Verification items for the finished model (mm, model axes). A direction names the side the tool comes from. Give positions to 0.01 mm unless a question says otherwise; leave off trailing zeros. Write each loop counter-clockwise with the first axis right and the second up, starting at its lowest first coordinate (ties: lowest second). Pieces come first, ordered by that corner, then holes. Notation, with made-up numbers: (12, 15) -> (31, 15) arc R24 cw to (31, 46) -> close; hole circle Ø11 at (71.5, 18). An arc over 180 degrees is marked (long way). Write item = value, one per line.
from build123d import *

# Parameters (mm, degrees)
SKETCH1_W           = 1043.686
SKETCH1_H           = 730.25
BOSS_EXTRUDE1_DEPTH = 6.35
SKETCH9_W           = 304.8
SKETCH9_H           = 304.8
CUT_EXTRUDE3_DEPTH  = 6.35
CUT_EXTRUDE4_DEPTH  = 6.35
FILLET1_R           = 6.35
CUT_EXTRUDE6_DEPTH  = 7.35


with BuildPart() as part:
    # Sketch1 → Boss-Extrude1 (new body)
    with BuildSketch(Plane.XY):
        with Locations((521.843, 365.125)):
            Rectangle(SKETCH1_W, SKETCH1_H)
    extrude(amount=BOSS_EXTRUDE1_DEPTH)

    # Sketch9 → Cut-Extrude3 (cut)
    with BuildSketch(Plane(origin=(0, 0, 0), x_dir=(-1, 0, 0), z_dir=(0, 0, -1))):
        with Locations((-196.85, 228.6)):
            Rectangle(SKETCH9_W, SKETCH9_H)
    extrude(amount=-CUT_EXTRUDE3_DEPTH, mode=Mode.SUBTRACT)

    # Sketch10 → Cut-Extrude4 (cut)
    with BuildSketch(Plane.XY.offset(6.35)):
        with BuildLine():
            Line((76.2, 50.8), (0, 50.8))
            Line((0, 50.8), (0, 0))
            Line((0, 0), (101.6, 0))
            Line((101.6, 0), (101.6, 25.4))
            ThreePointArc((101.6, 25.4), (94.160512242, 43.360512242), (76.2, 50.8))
        make_face()
        with BuildLine():
            Line((942.086, 25.4), (942.086, 0))
            Line((942.086, 0), (1043.686, 0))
            Line((1043.686, 0), (1043.686, 50.8))
            Line((1043.686, 50.8), (967.486, 50.8))
            ThreePointArc((967.486, 50.8), (949.525487758, 43.360512242), (942.086, 25.4))
        make_face()
        with BuildLine():
            Line((967.486, 558.8), (1043.686, 558.8))
            Line((1043.686, 558.8), (1043.686, 476.25))
            Line((1043.686, 476.25), (967.486, 476.25))
            ThreePointArc((967.486, 476.25), (949.525487758, 483.689487758), (942.086, 501.65))
            Line((942.086, 501.65), (942.086, 533.4))
            ThreePointArc((942.086, 533.4), (949.525487758, 551.360512242), (967.486, 558.8))
        make_face()
        with BuildLine():
            Line((76.2, 558.8), (0, 558.8))
            Line((0, 558.8), (0, 476.25))
            Line((0, 476.25), (76.2, 476.25))
            ThreePointArc((76.2, 476.25), (94.160512242, 483.689487758), (101.6, 501.65))
            Line((101.6, 501.65), (101.6, 533.4))
            ThreePointArc((101.6, 533.4), (94.160512242, 551.360512242), (76.2, 558.8))
        make_face()
        with BuildLine():
            Line((1043.686, 139.7), (1043.686, 165.1))
            Line((1043.686, 165.1), (992.886, 165.1))
            ThreePointArc((992.886, 165.1), (988.395871939, 163.240128061), (986.536, 158.75))
            Line((986.536, 158.75), (986.536, 146.05))
            ThreePointArc((986.536, 146.05), (988.395871939, 141.559871939), (992.886, 139.7))
            Line((992.886, 139.7), (1043.686, 139.7))
        make_face()
    extrude(amount=-CUT_EXTRUDE4_DEPTH, mode=Mode.SUBTRACT)

    # Fillet1
    fillet1_edges = [part.edges().sort_by_distance(p)[0] for p in [
        (349.25, 76.2, 3.175),
        (349.25, 381, 3.175),
        (44.45, 381, 3.175),
        (44.45, 76.2, 3.175),
        (1043.686, 558.8, 3.175),
        (1043.686, 476.25, 3.175),
        (1043.686, 50.8, 3.175),
        (942.086, 0, 3.175),
        (0, 476.25, 3.175),
        (0, 558.8, 3.175),
        (0, 730.25, 3.175),
        (1043.686, 730.25, 3.175),
        (1043.686, 139.7, 3.175),
        (1043.686, 165.1, 3.175),
        (101.6, 0, 3.175),
        (0, 50.8, 3.175),
    ]]
    fillet(fillet1_edges, radius=FILLET1_R)

    # Sketch14 → Cut-Extrude6 (cut, through all)
    with BuildSketch(Plane(origin=(0, 0, 0), x_dir=(-1, 0, 0), z_dir=(0, 0, -1))):
        with BuildLine():
            Line((-660.4, 692.15), (-254, 692.15))
            ThreePointArc((-254, 692.15), (-228.6, 666.75), (-254, 641.35))
            Line((-254, 641.35), (-660.4, 641.35))
            ThreePointArc((-660.4, 641.35), (-685.8, 666.75), (-660.4, 692.15))
        make_face()
    extrude(amount=-CUT_EXTRUDE6_DEPTH, mode=Mode.SUBTRACT)


solid = part.part
Item 1: Material ranges on line 1 (Y direction, x = 257.5, z = 4.5); line 2 (Y direction, x = 197, z = 3); line 3 (Y direction, x = 617.5, z = 2), recorded low to high.
Response values:
line_1 = 0 to 76.2, 381 to 641.35, 692.15 to 730.25
line_2 = 0 to 76.2, 381 to 730.25
line_3 = 0 to 641.35, 692.15 to 730.25
Item 2: Go/stop test with flat-tipped pins: P1, Ø3, axis at y = 17.5, z = 3, coming from the +X side; P2, Ø3, axis at x = 29.5, z = 1.5, coming from the -Y side. Record where each tip stops, or that it passes through.
Response values:
P1 = 942.09
P2 = 50.8
Item 3: Sectioned sample at C-C on z = 3. Give the number of separate pieces and of enclosed holes in the cut face, then the cut area to 3 significant figures.
Response values:
separate_pieces = 1
enclosed_holes = 2
area = 619,000 mm^2
Item 4: Sectioned sample at B-B on x = 554.5. Record the cut outline in (y, z).
Response values:
outline = (0, 0) -> (641.35, 0) -> (641.35, 6.35) -> (0, 6.35) -> close; (692.15, 0) -> (730.25, 0) -> (730.25, 6.35) -> (692.15, 6.35) -> close
Item 5: Sectioned sample at A-A on y = 666.75. Record the cut outline in (x, z).
Response values:
outline = (0, 0) -> (228.6, 0) -> (228.6, 6.35) -> (0, 6.35) -> close; (685.8, 0) -> (1043.69, 0) -> (1043.69, 6.35) -> (685.8, 6.35) -> close
Item 6: Mould release check, pull along X, two halves, no side actions. Record for faces 5 (the cylindrical face through (685.794, 666.191, 3.131)), 6 (the cylindrical face through (93.96, 483.49, 3.22)), 7 (the cylindrical face through (949.724, 483.493, 3.219)): +X half, -X half, draft (parallel to the pull), parting line (faces both ways), or undercut.
Response values:
face_5 = undercut
face_6 = -X half
face_7 = +X half
Item 7: Set-up check for faces 1 (the cylindrical face through (228.606, 667.309, 3.131)), 2 (the cylindrical face through (94.36, 551.16, 3.22)), 3 (the flat face through (631, 370, 6.35)), 4 (the cylindrical face through (949.329, 551.162, 3.219)): record each of +Z, -Z, +X, -X, +Y, -Y from which the full face is reachable in a straight line by a thin tool's end or side.
Response values:
face_1 = +Z, -Z
face_2 = +Z, -Z, -X
face_3 = +Z, +X, -X, +Y, -Y
face_4 = +Z, -Z, +X
